```python
from build123d import *

# Parameters (mm, degrees)
SKETCH2_R           = 10.5
SKETCH2_R_2         = 1.55
BOSS_EXTRUDE1_DEPTH = 4
SKETCH3_R           = 12
CUT_EXTRUDE1_DEPTH  = 2
CHAMFER1_SIZE       = 0.5


with BuildPart() as part:
    # Sketch2 → Boss-Extrude1 (new body)
    with BuildSketch(Plane.XY):
        with BuildLine():
            Line((-8.606779144, 16.938812023), (8.36334863, 17.060316518))
            ThreePointArc((8.36334863, 17.060316518), (18.999513009, 0.136034699), (8.606779144, -16.938812023))
            Line((8.606779144, -16.938812023), (-8.36334863, -17.060316518))
            ThreePointArc((-8.36334863, -17.060316518), (-18.999513009, -0.136034699), (-8.606779144, 16.938812023))
        make_face()
        with Locations((0, 0.289780582)):
            Circle(SKETCH2_R, mode=Mode.SUBTRACT)
        with Locations((-16, 0)):
            Circle(SKETCH2_R_2, mode=Mode.SUBTRACT)
        with Locations((-7.9995, 13.857272486)):
            Circle(SKETCH2_R_2, mode=Mode.SUBTRACT)
        with Locations((8.0015, 13.857272486)):
            Circle(SKETCH2_R_2, mode=Mode.SUBTRACT)
        with Locations((16.002, 0)):
            Circle(SKETCH2_R_2, mode=Mode.SUBTRACT)
        with Locations((8.0015, -13.857272486)):
            Circle(SKETCH2_R_2, mode=Mode.SUBTRACT)
        with Locations((-7.9995, -13.857272486)):
            Circle(SKETCH2_R_2, mode=Mode.SUBTRACT)
    extrude(amount=BOSS_EXTRUDE1_DEPTH)

    # Sketch3 → Cut-Extrude1 (cut)
    with BuildSketch(Plane.XY.offset(4)):
        Circle(SKETCH3_R)
    extrude(amount=-CUT_EXTRUDE1_DEPTH, mode=Mode.SUBTRACT)

    # Chamfer1
    chamfer1_edges = [part.edges().sort_by_distance(p)[0] for p in [
        (18.999513009, 0.136034699, 4),
        (-10.5, 0.289780582, 2),
        (-12, 0, 4),
        (-18.999513009, -0.136034699, 4),
        (18.999513009, 0.136034699, 0),
        (-18.999513009, -0.136034699, 0),
    ]]
    chamfer(chamfer1_edges, length=CHAMFER1_SIZE)


solid = part.part
```
Could you check a few things on this model? Use its own coordinates, in mm. A direction names the side the tool comes from. Coordinates: 2 decimals unless noted, no trailing zeros. Loops run counter-clockwise (first coordinate to the right, second up) from the corner with the lowest first, then second, coordinate; pieces in that order, holes last.
1) Imagine slicing it at A-A (x = 0). List the corners of the cut face in (y, z) for me, and give its area (3 significant figures).
Reported:
outline: (-17, 0) - (-10.21, 0) - (-10.21, 1.5) - (-10.71, 2) - (-12, 2) - (-12, 3.5) - (-12.5, 4) - (-17, 4) - close; (10.79, 0) - (17, 0) - (17, 4) - (12.5, 4) - (12, 3.5) - (12, 2) - (11.29, 2) - (10.79, 1.5) - close
area: 45.5 mm2
2) Please list where these lines run through material, in increasing order: line 1 along Y through (x, z) = (9, 1.85); line 2 along X through (y, z) = (-14.5, 2.3); line 3 along Y through (x, z) = (-8.5, 2.2).
Reported:
line 1: y = -16.73 to -15.04, -12.67 to -5.77, 6.35 to 12.67, 15.04 to 16.73
line 2: x = -12.28 to -9.41, -6.59 to 6.59, 9.41 to 12.28
line 3: y = -16.99 to -15.32, -12.39 to -8.47, 8.47 to 12.39, 15.32 to 16.94
3) Will these pins go through, and if not, where does the flat tip stop? pin 1 Ø19 at (x, y) = (0, 0.29) entering from +Z; pin 2 Ø1.5 at (x, y) = (-11.5, 4) entering from -Z; pin 3 Ø2 at (y, z) = (11, 2.5) entering from +X; pin 4 Ø2 at (y, z) = (12, 0.5) entering from +X.
Reported:
pin 1: passes through
pin 2: stops at z = 0
pin 3: stops at x = 16.16
pin 4: stops at x = 15.49
4) Imagine slicing it at B-B (z = 2.7). List the corners of the cut face in (x, y) for me, and give its area (3 significant figures).
Reported:
outline: (-8.61, 16.94) arc R19 ccw to (-8.36, -17.06) - (8.61, -16.94) arc R19 ccw to (8.36, 17.06) - close; hole circle Ø3.1 at (-16, 0); hole circle Ø24 at (0, 0); hole circle Ø3.1 at (-8, -13.86); hole circle Ø3.1 at (-8, 13.86); hole circle Ø3.1 at (8, -13.86); hole circle Ø3.1 at (8, 13.86); hole circle Ø3.1 at (16, 0)
area: 591 mm2
5) Which directions (+Z, -Z, +X, -X, +Y, -Y) give clear straight access to the entire face, cutting with the end or side of a thin tool? Please do faces 4 (the face through (2, -11, 2)), 5 (the face through (-17.55, 0.07, 1.97)).
Reported:
face 4: +Z
face 5: +Z, -Z
6) Thinking about a two-plate mould opening in X: for faces 1 (the face through (-7.284, 12.482, 1.972)), 2 (the face through (8, 8, 0)), 3 (the face through (-18.63, -0.437, 0.135)), which applies, released by +X, released by -X, zero draft, split by the parting line, or undercut?
Reported:
face 1: undercut
face 2: zero draft
face 3: released by -X
